```python
from build123d import *

# Parameters (mm, degrees)
F0_W     = 8.5
F0_H     = 26
F1_DEPTH = 4.25
F5_DEPTH = 4


with BuildPart() as f1:
    # F0 (on Top) → F1 (new body, symmetric)
    with BuildSketch(Plane.XY):
        with Locations((0, 13)):
            Rectangle(F0_W, F0_H)
    extrude(amount=F1_DEPTH, both=True)

    # F2 (on Right) → F3 (revolve, cut)
    with BuildSketch(Plane.YZ):
        Polygon((23.7, 3.95), (23.5, 4.25), (21.7, 4.25), (21.7, 0.35), (23.7, 0.35), align=None)
    revolve(axis=Axis((0, 21.7, 2.3), (0, 0, 1)), mode=Mode.SUBTRACT)

    # F4 (on face) → F5 (cut)
    with BuildSketch(Plane.XY.offset(4.25)):
        Polygon((-3.75, 6), (-4.25, 6.5), (-4.25, 2.5), (-3.75, 3), (-2.5, 2), (-1.25, 3), (0, 2), (1.25, 3), (2.5, 2), (3.75, 3), (4.25, 2.5), (4.25, 6.5), (3.75, 6), (2.5, 7), (1.25, 6), (0, 7), (-1.25, 6), (-2.5, 7), align=None)
    extrude(amount=-F5_DEPTH, mode=Mode.SUBTRACT)


solid = f1.part
```
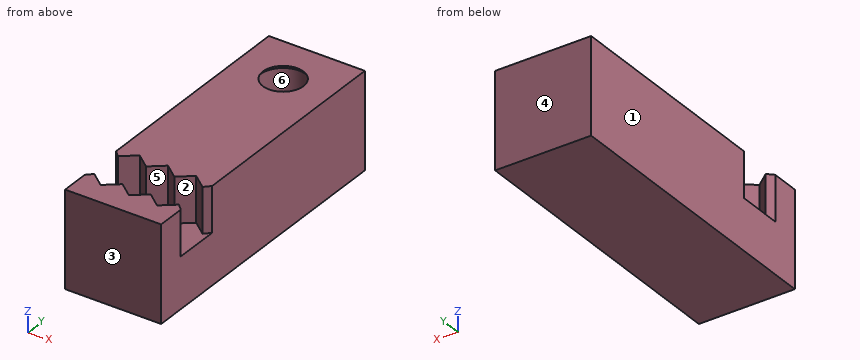
Design review of the part built by this model. Coordinates are the model's own, in mm. Face numbers are marked on the shaded views. A direction names the side the tool comes from. Round coordinates to 2 decimals unless told otherwise and drop trailing zeros. Order: outer loops, then holes, each group sorted by start corner. A loop starts at its lowest first (then second) coordinate and runs counter-clockwise, first axis right, second up. Notation, with made-up numbers: (-7, 12) - (2, 12) arc R15 cw to (2, 31) - close; hole circle Ø2 at (69, 82.25). An arc over 180 degrees is marked (long way). Return JSON: item names as keys, results as strings.
Q1. The part is to be moulded in two halves that separate along Y. For the marked faces 3, 4, 5 and 6, say which applies: pulls with the +Y half, pulls with the -Y half, needs draft (parallel to the pull), parting line crosses it, or undercut.
Computed values:
{"face 3": "pulls with the -Y half", "face 4": "pulls with the +Y half", "face 5": "undercut", "face 6": "undercut"}
Q2. Consider section D-D on x = -3. Write out the cut boundary in (y, z).
Computed values:
{"outline": "(0, -4.25) - (26, -4.25) - (26, 4.25) - (6.6, 4.25) - (6.6, 0.25) - (2.4, 0.25) - (2.4, 4.25) - (0, 4.25) - close"}
Q3. Consider section C-C on y = 21.7. Write out the cut boundary in (x, z).
Computed values:
{"outline": "(-4.25, -4.25) - (4.25, -4.25) - (4.25, 4.25) - (1.8, 4.25) - (2, 3.95) - (2, 0.35) - (-2, 0.35) - (-2, 3.95) - (-1.8, 4.25) - (-4.25, 4.25) - close"}
Q4. Consider section A-A on z = 1. Write out the cut boundary in (x, y).
Computed values:
{"outline": "(-4.25, 0) - (4.25, 0) - (4.25, 2.5) - (3.75, 3) - (2.5, 2) - (1.25, 3) - (0, 2) - (-1.25, 3) - (-2.5, 2) - (-3.75, 3) - (-4.25, 2.5) - close; (-4.25, 6.5) - (-3.75, 6) - (-2.5, 7) - (-1.25, 6) - (0, 7) - (1.25, 6) - (2.5, 7) - (3.75, 6) - (4.25, 6.5) - (4.25, 26) - (-4.25, 26) - close; hole circle Ø4 at (0, 21.7)"}
Q5. Consider section B-B on x = 2.25. Write out the cut boundary in (y, z).
Computed values:
{"outline": "(0, -4.25) - (26, -4.25) - (26, 4.25) - (6.8, 4.25) - (6.8, 0.25) - (2.2, 0.25) - (2.2, 4.25) - (0, 4.25) - close"}
Q6. Wall thickness on L1, parallel to X at y = 21.7, z = 1.45; L2, parallel to Z at x = -0.5, y = 21; L3, parallel to Z at x = 3, y = 4: over which ranges is each line inside the solid? List them lowest first. Write a range as [from, to].
Computed values:
{"L1": "x = [-4.25, -2], [2, 4.25]", "L2": "z = [-4.25, 0.35]", "L3": "z = [-4.25, 0.25]"}
Q7. Machinability: for the marked faces 1 and 2, which of the approach directions +Z, -Z, +X, -X, +Y, -Y give a long, thin tool a straight path to every point of the face, cutting with its end or side? Answer none if there is none.
Computed values:
{"face 1": "+Z, -Z, -X, +Y, -Y", "face 2": "+Z"}
